Design review of the part built by this model. Coordinates are the model's own, in mm. Face numbers are marked on the shaded views. Round coordinates to 2 decimals unless told otherwise and drop trailing zeros. Loops run counter-clockwise (first coordinate to the right, second up) from the corner with the lowest first, then second, coordinate; pieces in that order, holes last. Notation, with made-up numbers: (-4, 64.25) - (38, 64.25) arc R22 cw to (38, 99.25) - close; hole circle Ø8 at (10.25, 60). An arc over 180 degrees is marked (long way). Use one line per item in the form item = value. Start each with the question number.
(1) The part is to be moulded in two halves that separate along Y. For the marked faces 1, 2, 3 and 4, say which applies: released by +Y, released by -Y, zero draft, split by the parting line, or undercut.
(2) Wall thickness on probe 1 along X at (y, z) = (10, -103.5); probe 2 along Y at (x, z) = (0, -126) (3 decimals); probe 3 along X at (y, z) = (-10.5, -104): over which ranges is each line inside the solid? List them lowest first. Write a range as [from, to].
(3) We need section B-B, the plane z = -77.5. Write out the cut boundary in (x, y).
(4) For pin 1 (5 mm diameter, centred on y = -6.5, z = -85.5, fed in from -X); pin 2 (12 mm diameter, centred on y = -5, z = -126, fed in from -X); pin 3 (2 mm diameter, centred on x = 22, y = 20, fed in from -Z), all flat-tipped, find the tip position at first contact; note any pin that passes through.
(5) We need section A-A, the plane z = -121.5. Write out the cut boundary in (x, y) (3 decimals).
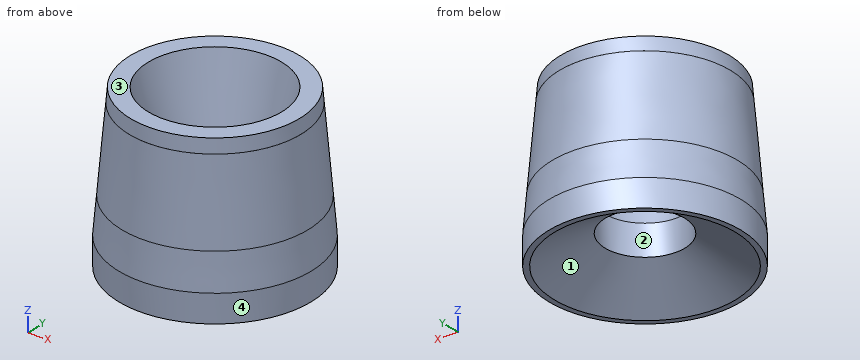
from build123d import *


with BuildPart() as part:
    # Sketch1 → Revolve1 (revolve)
    with BuildSketch(Plane(origin=(0, 0, 0), x_dir=(1, 0, 0), z_dir=(0, 1, 0)), mode=Mode.PRIVATE) as revolve1_sk:
        Polygon((44.323, 130.833403353), (44.323, 143.454534929), (18.415, 128.496544155), (18.415, 120.876544155), (32.087521299, 69.85), (38.987643543, 69.85), (39.543196557, 76.2), (39.544164949, 76.211068779), (42.87748303, 114.311068779), align=None)
    revolve(revolve1_sk.sketch.rotate(Axis((0, 0, -146.817261676), (0, 0, 1)), 180), axis=Axis((0, 0, -146.817261676), (0, 0, 1)))

    # Sketch2 → Revolve2 (revolve)
    with BuildSketch(Plane(origin=(0, 0, 0), x_dir=(1, 0, 0), z_dir=(0, 1, 0)), mode=Mode.PRIVATE) as revolve2_sk:
        Polygon((18.415, 120.876544155), (18.415, 115.969640957), (30.77272055, 69.85), (32.087521299, 69.85), align=None)
        Polygon((18.415, 129.963013839), (41.783, 143.454534929), (44.323, 143.454534929), (18.415, 128.496544155), align=None)
    revolve(revolve2_sk.sketch.rotate(Axis((0, 0, -146.817261676), (0, 0, 1)), 180), axis=Axis((0, 0, -146.817261676), (0, 0, 1)))


solid = part.part
Data:
q1.face_1 = undercut
q1.face_2 = undercut
q1.face_3 = zero draft
q1.face_4 = split by the parting line
q2.probe_1 = [-40.72, -19.32], [19.32, 40.72]
q2.probe_2 = [-43.9, -18.415], [18.415, 43.9]
q2.probe_3 = [-40.64, -18.9], [18.9, 40.64]
q3.outline = circle Ø79.31 at (0, 0); hole circle Ø57.45 at (0, 0)
q4.pin_1 = -40.24
q4.pin_2 = -44.3
q4.pin_3 = -137.07
q5.outline = circle Ø87.013 at (0, 0); hole circle Ø36.83 at (0, 0)
